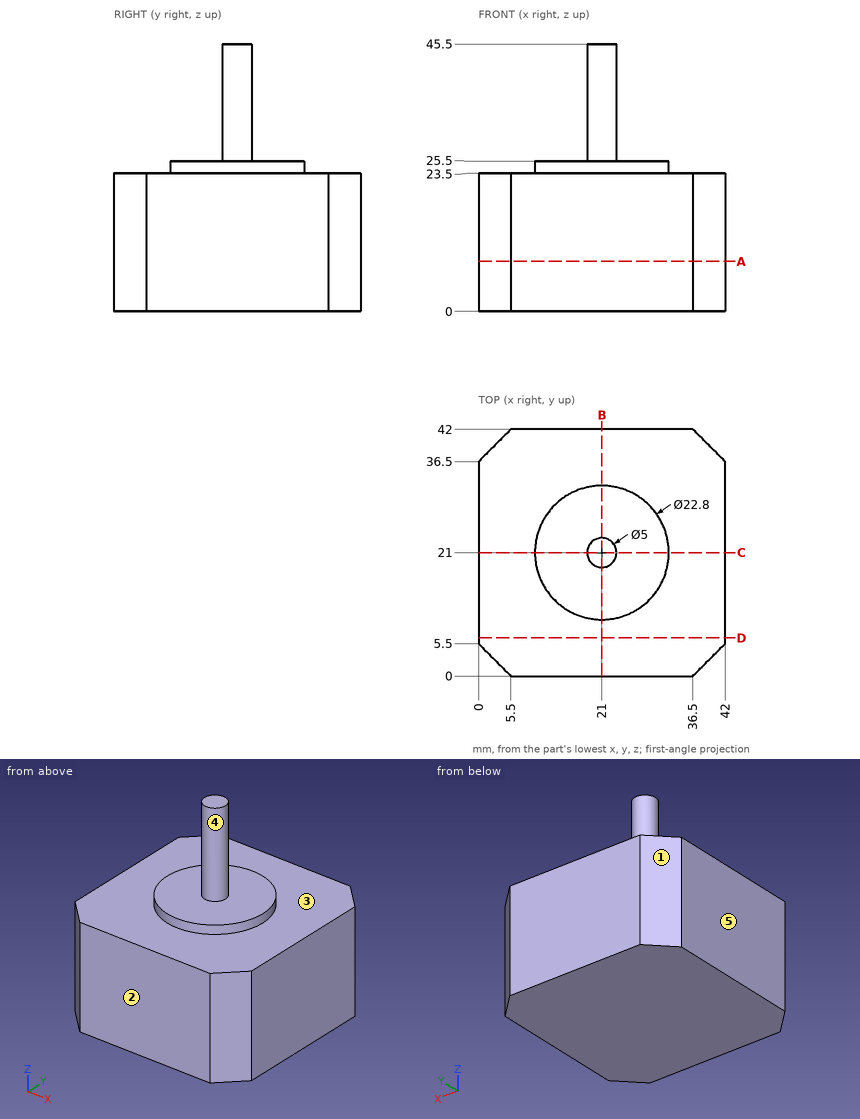
Geometry check sheet. Reference: drawing and pictorial views, mm from the part's lowest x, y, z. A direction names the side the tool comes from. Round coordinates to 2 decimals unless told otherwise and drop trailing zeros. Order: outer loops, then holes, each group sorted by start corner. A loop starts at its lowest first (then second) coordinate and runs counter-clockwise, first axis right, second up. Notation, with made-up numbers: (-34, -38.5) - (-13, -38.5) arc R15 cw to (-13, -19.5) - close; hole circle Ø2 at (-26, 72). An arc over 180 degrees is marked (long way). One line per question, with ' | ' between items. Start each with the question number.
(1) Release check for a two-part mould opening along Y. For the marked faces 1, 2 and 3 record: released by +Y, released by -Y, zero draft, split by the parting line, or undercut.
(2) Sectioned sample at D-D on y = 6.5. Record the cut outline in (x, z), and give its area (3 significant figures).
(3) Sectioned sample at A-A on z = 8.5. Record the cut outline in (x, y).
(4) Thickness scan on L1, parallel to Z at x = 4, y = 24; L2, parallel to Z at x = 18, y = 19.5. Record the ranges inside material, lowest first. Write a range as [from, to].
(5) Sectioned sample at B-B on x = 21. Record the cut outline in (y, z), and give its area (3 significant figures).
(6) Access from +Z, -Z, +X, -X, +Y, -Y to the whole of each face (thin tool, end or side, straight path). Record for the marked faces 4 and 5.
(7) Depth check by flat-ended pin: pin 1 Ø25 at (x, y) = (24.5, 19) entering from +Z; pin 2 Ø5 at (y, z) = (15, 35.5) entering from +X; pin 3 Ø1.5 at (x, y) = (33, 12) entering from +Z; pin 4 Ø4 at (y, z) = (12.5, 26.5) entering from +X. Enter the tip coordinate at first touch or a pass-through.
Conclusion:
1) face 1: released by +Y | face 2: released by -Y | face 3: zero draft
2) outline: (0, 0) - (42, 0) - (42, 23.5) - (0, 23.5) - close | area: 987 mm2
3) outline: (0, 5.5) - (5.5, 0) - (36.5, 0) - (42, 5.5) - (42, 36.5) - (36.5, 42) - (5.5, 42) - (0, 36.5) - close
4) L1: z = [0, 23.5] | L2: z = [0, 25.5]
5) outline: (0, 0) - (42, 0) - (42, 23.5) - (32.4, 23.5) - (32.4, 25.5) - (23.5, 25.5) - (23.5, 45.5) - (18.5, 45.5) - (18.5, 25.5) - (9.6, 25.5) - (9.6, 23.5) - (0, 23.5) - close | area: 1,130 mm2
6) face 4: +Z | face 5: +Z, -Z, -X, +Y, -Y
7) pin 1: stops at z = 45.5 | pin 2: passes through | pin 3: stops at z = 23.5 | pin 4: stops at x = 30.17
